from build123d import *

# Parameters (mm, degrees)
F1_DEPTH = 3.3


with BuildPart() as f1:
    # F0 (on Top) → F1 (new body)
    with BuildSketch(Plane.XY):
        with BuildLine():
            ThreePointArc((0, 1.5), (0.43934, 0.43934), (1.5, 0))
            Line((1.5, 0), (23.5, 0))
            ThreePointArc((23.5, 0), (24.56066, 0.43934), (25, 1.5))
            ThreePointArc((25, 1.5), (24.56066, 2.56066), (23.5, 3))
            Line((23.5, 3), (1.5, 3))
            ThreePointArc((1.5, 3), (0.43934, 2.56066), (0, 1.5))
        make_face()
    extrude(amount=F1_DEPTH)


solid = f1.part
Build history of the part. All positions in model axes, mm. Round coordinates to 2 decimals unless told otherwise and drop trailing zeros. Write each loop counter-clockwise with the first axis right and the second up, starting at its lowest first coordinate (ties: lowest second). Pieces come first, ordered by that corner, then holes. Notation, with made-up numbers: (-11, 33) - (6, 33) arc R31 ccw to (6, 59) - close; hole circle Ø3 at (11.25, 26.25). An arc over 180 degrees is marked (long way). Use CSV: the item, a comma, the result in double quotes.
(1) Band-saw the part on B-B (y = 2.4). Write the cut outline in (x, z).
Response:
outline,"(0.3, 0) - (24.7, 0) - (24.7, 3.3) - (0.3, 3.3) - close"
(2) Band-saw the part on A-A (z = 0.65). Write the cut outline in (x, y), plus the area to 3 significant figures.
Response:
outline,"(0, 1.5) arc R1.5 ccw to (1.5, 0) - (23.5, 0) arc R1.5 ccw to (25, 1.5) arc R1.5 ccw to (23.5, 3) - (1.5, 3) arc R1.5 ccw to start"
area,"73.1 mm²"
(3) Wall check: line 1 (X direction, y = 0.55, z = 2.6); line 2 (X direction, y = 0.2, z = 2.35). Give the ranges that are in metal, low to high.
Response:
line 1,"0.34 to 24.66"
line 2,"0.75 to 24.25"
